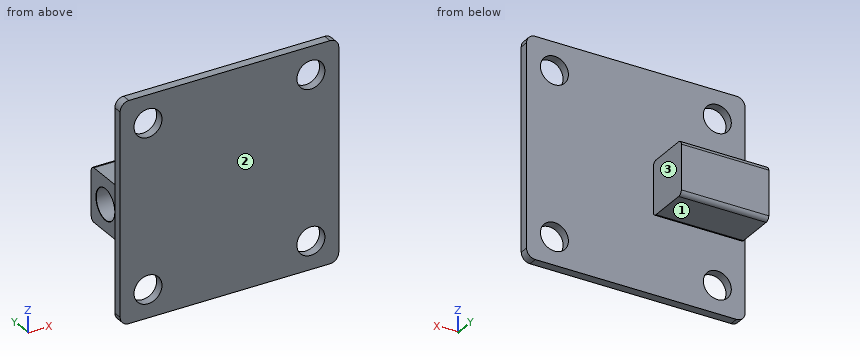
```python
from build123d import *

# Parameters (mm, degrees)
SKETCH_2_W                        = 25
SKETCH_2_H                        = 25
SKETCH_2_R                        = 1.6
EXTRUDE_1_DEPTH                   = 1
FILLET_1_R                        = 1
EXTRUDE_START                     = -0.5
EXTRUDE_2_DEPTH                   = 10
HOLE_WIZARD_3_5_3_5_1_D           = 3.5
HOLE_WIZARD_3_5_3_5_1_DEPTH       = 6
HOLE_WIZARD_3_5_3_5_1_CSINK_D     = 3.55
HOLE_WIZARD_3_5_3_5_1_CSINK_ANGLE = 90
HOLE_WIZARD_3_5_3_5_1_TIP         = 1.051506083


with BuildPart() as part:
    # 스케치2 → 보스-돌출1 (new body)
    with BuildSketch(Plane(origin=(0, 0, 0), x_dir=(1, 0, 0), z_dir=(0, 1, 0))):
        with Locations((-28.42313588, -14.815)):
            Rectangle(SKETCH_2_W, SKETCH_2_H)
        with Locations(Location((-19.11, -24.13, 0), (0, 0, 270))):
            Circle(SKETCH_2_R, mode=Mode.SUBTRACT)
        with Locations(Location((-37.73627176, -24.13, 0), (0, 0, 270))):
            Circle(SKETCH_2_R, mode=Mode.SUBTRACT)
        with Locations(Location((-37.73627176, -5.5, 0), (0, 0, 270))):
            Circle(SKETCH_2_R, mode=Mode.SUBTRACT)
        with Locations(Location((-19.11, -5.5, 0), (0, 0, 270))):
            Circle(SKETCH_2_R, mode=Mode.SUBTRACT)
    extrude(amount=EXTRUDE_1_DEPTH)

    # 필렛1
    fillet_1_edges = [part.edges().sort_by_distance(p)[0] for p in [
        (-15.92313588, 0.5, 27.315),
        (-40.92313588, 0.5, 27.315),
        (-40.92313588, 0.5, 2.315),
        (-15.92313588, 0.5, 2.315),
    ]]
    fillet(fillet_1_edges, radius=FILLET_1_R)

    # 스케치4 → 보스-돌출2 (add)
    with BuildSketch(Plane.ZY.offset(40.92313588).offset(EXTRUDE_START)):
        with BuildLine():
            Line((11.536225379, 1), (16.659931287, 1))
            ThreePointArc((16.659931287, 1), (17.013484677, 1.146446609), (17.159931287, 1.5))
            Line((17.159931287, 1.5), (17.159931287, 5.75777714))
            ThreePointArc((17.159931287, 5.75777714), (17.013484677, 6.111330531), (16.659931287, 6.25777714))
            Line((16.659931287, 6.25777714), (11.536225379, 6.25777714))
            ThreePointArc((11.536225379, 6.25777714), (11.182671988, 6.111330531), (11.036225379, 5.75777714))
            Line((11.036225379, 5.75777714), (11.036225379, 1.5))
            ThreePointArc((11.036225379, 1.5), (11.182671988, 1.146446609), (11.536225379, 1))
        make_face()
    extrude(amount=-EXTRUDE_2_DEPTH)

    # Ø3.5 (3.5) 지름 구멍1
    with Locations(Plane.ZY.offset(40.42313588)):
        with Locations((14.083142465, 3.599368414)):
            CounterSinkHole(HOLE_WIZARD_3_5_3_5_1_D / 2, HOLE_WIZARD_3_5_3_5_1_CSINK_D / 2, depth=HOLE_WIZARD_3_5_3_5_1_DEPTH, counter_sink_angle=HOLE_WIZARD_3_5_3_5_1_CSINK_ANGLE)
            with Locations((0, 0, -(HOLE_WIZARD_3_5_3_5_1_DEPTH + HOLE_WIZARD_3_5_3_5_1_TIP / 2))):  # 118° drill point
                Cone(0, HOLE_WIZARD_3_5_3_5_1_D / 2, HOLE_WIZARD_3_5_3_5_1_TIP, mode=Mode.SUBTRACT)


solid = part.part
```
Check sheet for the modelled part. Datum: model origin and axes. Units: mm. Face numbers are marked on the shaded views. A direction names the side the tool comes from. Round coordinates to 2 decimals unless told otherwise and drop trailing zeros. Write each loop counter-clockwise with the first axis right and the second up, starting at its lowest first coordinate (ties: lowest second). Pieces come first, ordered by that corner, then holes. Notation, with made-up numbers: M 43,-11.75 L 74,-11.75 A32 ccw 74,19.25 Z; hole C -38.5,18.25 d5. An arc over 180 degrees is marked long. Write item = value, one per line. Start each with the question number.
1. Gauge pin test, flat ends, axial feed: pin 1 (6 mm diameter, centred on x = -31, z = 20, fed in from +Y); pin 2 (4 mm diameter, centred on x = -19.11, z = 5.5, fed in from +Y); pin 3 (2.5 mm diameter, centred on y = 3, z = 13.5, fed in from -X); pin 4 (2.5 mm diameter, centred on x = -37.74, z = 5.5, fed in from +Y). Record the tip position at first contact, or that the pin passes through.
2. Tool access check on the marked faces 1, 2 and 3. Record the directions out of +Z, -Z, +X, -X, +Y, -Y that give a thin tool (end or side, any length) a straight path to the whole face; none if there is none.
3. Section check C-C, the plane x = -36.5. Record the cut outline in (y, z) (3 decimals), then the cut area to 3 significant figures.
4. Scan lines: line 1 (X direction, y = 0.45, z = 5.5); line 2 (Z direction, x = -31.75, y = 2.75); line 3 (Y direction, x = -24.25, z = 10.5). Record each from-to range of solid material in increasing order. Write a range as [from, to].
5. Section check A-A, the plane z = 24.13. Record the cut outline in (x, y), then the cut area to 3 significant figures.
6. Section check B-B, the plane x = -19.11. Record the cut outline in (y, z) (3 decimals).
7. Section check D-D, the plane z = 19.5. Record the cut outline in (x, y).
Results found:
q1.pin_1 = 6.12
q1.pin_2 = 1
q1.pin_3 = -40.42
q1.pin_4 = through
q2.face_1 = -Z, +X, -X, +Y
q2.face_2 = +Z, -Z, +X, -X, -Y
q2.face_3 = +Z, -Z, +X, +Y
q3.outline = M 0,2.315 L 1,2.315 L 1,4.484 L 0,4.484 Z; M 0,6.516 L 1,6.516 L 1,11.536 A0.5 ccw 1.5,11.036 L 5.758,11.036 A0.5 ccw 6.258,11.536 L 6.258,16.66 A0.5 ccw 5.758,17.16 L 1.5,17.16 A0.5 ccw 1,16.66 L 1,23.114 L 0,23.114 Z; M 0,25.146 L 1,25.146 L 1,27.315 L 0,27.315 Z; hole C 3.599,14.083 d3.5
q3.area = 43.3 mm^2
q4.line_1 = [-40.92, -39.34], [-36.14, -20.71], [-17.51, -15.92]
q4.line_2 = [11.04, 17.16]
q4.line_3 = [0, 1]
q5.outline = M -40.92,0 L -39.34,0 L -39.34,1 L -40.92,1 Z; M -36.14,0 L -20.71,0 L -20.71,1 L -36.14,1 Z; M -17.51,0 L -15.92,0 L -15.92,1 L -17.51,1 Z
q5.area = 18.6 mm^2
q6.outline = M 0,2.315 L 1,2.315 L 1,3.9 L 0,3.9 Z; M 0,7.1 L 1,7.1 L 1,22.53 L 0,22.53 Z; M 0,25.73 L 1,25.73 L 1,27.315 L 0,27.315 Z
q7.outline = M -40.92,0 L -15.92,0 L -15.92,1 L -40.92,1 Z
